Part model, mm, in its own coordinate system. Face numbers are marked on the shaded views. A direction names the side the tool comes from. Coordinates: 2 decimals unless noted, no trailing zeros. Write each loop counter-clockwise with the first axis right and the second up, starting at its lowest first coordinate (ties: lowest second). Pieces come first, ordered by that corner, then holes. Notation, with made-up numbers: (76.5, 14.25) -> (92.5, 14.25) arc R10 cw to (92.5, 26.25) -> close; hole circle Ø4 at (75.5, 17). An arc over 180 degrees is marked (long way). Write item = value, one per line.
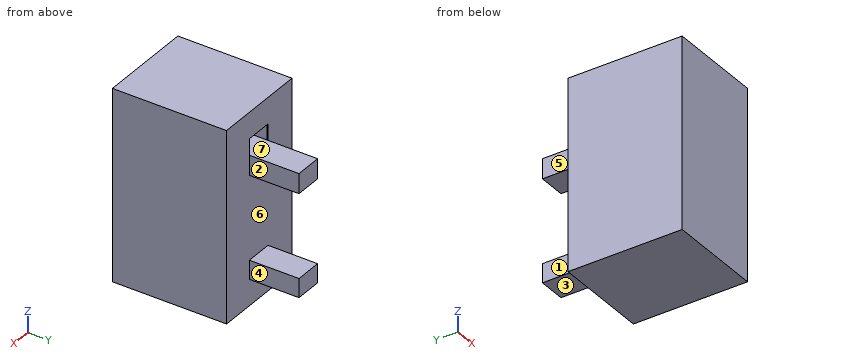
from build123d import *

# Parameters (mm, degrees)
ESQUISSE2_W             = 510
ESQUISSE2_H             = 1010
BOSS_EXTRU_1_DEPTH      = 5
ESQUISSE4_W             = 510
ESQUISSE4_H             = 1010
ESQUISSE4_W_2           = 500
ESQUISSE4_H_2           = 1000
BOSS_EXTRU_2_DEPTH      = 595
ESQUISSE5_W             = 510
ESQUISSE5_H             = 1010
BOSS_EXTRU_3_DEPTH      = 5
ESQUISSE6_W             = 145
ESQUISSE6_H             = 191
ESQUISSE6_H_2           = 100
ENL_V_MAT_EXTRU_1_DEPTH = 10
ESQUISSE8_W             = 145
ESQUISSE8_H             = 100
ESQUISSE8_H_2           = 105
BOSS_EXTRU_5_DEPTH      = 863


with BuildPart() as part:
    # Esquisse2 → Boss.-Extru.1 (new body)
    with BuildSketch(Plane(origin=(0, 0, 0), x_dir=(1, 0, 0), z_dir=(0, 1, 0))):
        with Locations((199.263257584, -405.525758022)):
            Rectangle(ESQUISSE2_W, ESQUISSE2_H)
    extrude(amount=BOSS_EXTRU_1_DEPTH)

    # Esquisse4 → Boss.-Extru.2 (add)
    with BuildSketch(Plane(origin=(0, 5, 0), x_dir=(1, 0, 0), z_dir=(0, 1, 0))):
        with Locations((199.263257584, -405.525758022)):
            Rectangle(ESQUISSE4_W, ESQUISSE4_H)
        with Locations((199.263257584, -405.525758022)):
            Rectangle(ESQUISSE4_W_2, ESQUISSE4_H_2, mode=Mode.SUBTRACT)
    extrude(amount=BOSS_EXTRU_2_DEPTH)

    # Esquisse5 → Boss.-Extru.3 (add)
    with BuildSketch(Plane(origin=(0, 600, 0), x_dir=(1, 0, 0), z_dir=(0, 1, 0))):
        with Locations((199.263257584, -405.525758022)):
            Rectangle(ESQUISSE5_W, ESQUISSE5_H)
    extrude(amount=BOSS_EXTRU_3_DEPTH)

    # Esquisse6 → Enlèv. mat.-Extru.1 (cut)
    with BuildSketch(Plane(origin=(0, 605, 0), x_dir=(1, 0, 0), z_dir=(0, 1, 0))):
        with Locations((204.263257584, -677.025758022)):
            Rectangle(ESQUISSE6_W, ESQUISSE6_H)
        with Locations((204.263257584, -88.525758022)):
            Rectangle(ESQUISSE6_W, ESQUISSE6_H_2)
    extrude(amount=-ENL_V_MAT_EXTRU_1_DEPTH, mode=Mode.SUBTRACT)

    # Esquisse8 → Boss.-Extru.5 (add)
    with BuildSketch(Plane(origin=(0, 5, 0), x_dir=(1, 0, 0), z_dir=(0, 1, 0))):
        with Locations((204.263257584, -88.525758022)):
            Rectangle(ESQUISSE8_W, ESQUISSE8_H)
        with Locations((204.263257584, -634.025758022)):
            Rectangle(ESQUISSE8_W, ESQUISSE8_H_2)
    extrude(amount=BOSS_EXTRU_5_DEPTH)


solid = part.part
Q1. Saw through at D-D on y = 709. Give the cut face in (x, z), and give its area (3 significant figures).
Model answer:
outline = (131.76, 38.53) -> (276.76, 38.53) -> (276.76, 138.53) -> (131.76, 138.53) -> close; (131.76, 581.53) -> (276.76, 581.53) -> (276.76, 686.53) -> (131.76, 686.53) -> close
area = 29,700 mm²
Q2. Probe line 1 (Z direction, x = 268.5, y = 352); line 2 (X direction, y = 563, z = 26); line 3 (Y direction, x = 53, z = -21.5). List the from-to ranges inside material, lowest first. Write a range as from..to.
Model answer:
line_1 = -99.47..-94.47, 38.53..138.53, 581.53..686.53, 905.53..910.53
line_2 = -55.74..-50.74, 449.26..454.26
line_3 = 0..5, 600..605
Q3. Saw through at A-A on z = 124.5. Give the cut face in (x, y), and give its area (3 significant figures).
Model answer:
outline = (-55.74, 0) -> (454.26, 0) -> (454.26, 605) -> (276.76, 605) -> (276.76, 868) -> (131.76, 868) -> (131.76, 605) -> (-55.74, 605) -> close; hole (-50.74, 5) -> (131.76, 5) -> (131.76, 600) -> (-50.74, 600) -> close; hole (276.76, 5) -> (449.26, 5) -> (449.26, 600) -> (276.76, 600) -> close
area = 135,000 mm²
Q4. Saw through at C-C on x = 221. Give the cut face in (y, z).
Model answer:
outline = (0, -99.47) -> (605, -99.47) -> (605, 38.53) -> (868, 38.53) -> (868, 138.53) -> (605, 138.53) -> (605, 581.53) -> (868, 581.53) -> (868, 686.53) -> (5, 686.53) -> (5, 905.53) -> (600, 905.53) -> (600, 772.53) -> (605, 772.53) -> (605, 910.53) -> (0, 910.53) -> close; hole (5, -94.47) -> (600, -94.47) -> (600, 38.53) -> (5, 38.53) -> close; hole (5, 138.53) -> (600, 138.53) -> (600, 581.53) -> (5, 581.53) -> close
Q5. Pin check, flat tip, straight feed: pin 1 (5 mm diameter, centred on x = 287.5, z = 382, fed in from +Y). Stop position of the tip, or through.
Model answer:
pin_1 = 605
Q6. Mould opens along X. For the marked faces 4, 5, 6 and 7 say: released by +X, released by -X, zero draft, split by the parting line, or undercut.
Model answer:
face_4 = released by +X
face_5 = released by -X
face_6 = zero draft
face_7 = undercut
Q7. Which spindle directions (+Z, -Z, +X, -X, +Y, -Y) get a long thin tool onto all of the face, cutting with end or side? Do the marked faces 1, 2 and 3. Say none if no direction does.
Model answer:
face_1 = +Z, -Z, -X, +Y
face_2 = +Z, -Z, +X, +Y
face_3 = -Z, +X, -X, +Y
Q8. Saw through at B-B on y = 295.5. Give the cut face in (x, z).
Model answer:
outline = (-55.74, -99.47) -> (454.26, -99.47) -> (454.26, 910.53) -> (-55.74, 910.53) -> close; (131.76, 38.53) -> (276.76, 38.53) -> (276.76, 138.53) -> (131.76, 138.53) -> close; (131.76, 581.53) -> (276.76, 581.53) -> (276.76, 686.53) -> (131.76, 686.53) -> close; hole (-50.74, -94.47) -> (449.26, -94.47) -> (449.26, 905.53) -> (-50.74, 905.53) -> close
